Model file for the job. Use its own axes, mm. Face numbers are marked on the shaded views. A direction names the side the tool comes from. Coordinates: 2 decimals unless noted, no trailing zeros. Loops run counter-clockwise (first coordinate to the right, second up) from the corner with the lowest first, then second, coordinate; pieces in that order, holes last. Notation, with made-up numbers: (72, -24) -> (91, -24) arc R22 ccw to (91, -2) -> close; hole circle Ø8 at (88, 46). An arc over 180 degrees is marked (long way). Use one line per item in the form item = value.
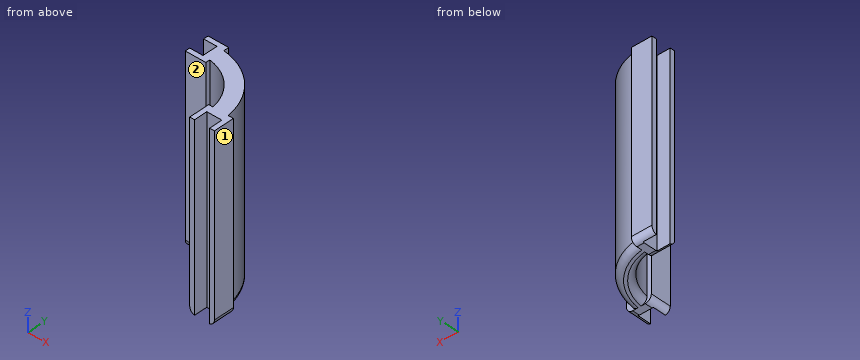
```python
from build123d import *

# Parameters (mm, degrees)
EXTRUDE_1_DEPTH = 150
EXTRUDE_2_DEPTH = 150
FILLET_1_R      = 5
FILLET_2_R      = 5
FILLET_3_R      = 5
FILLET_4_R      = 5
FILLET_5_R      = 5


with BuildPart() as part:
    # 草图1 → 凸台-拉伸1 (new body)
    with BuildSketch(Plane.XY):
        with BuildLine():
            Line((0, 40), (0, 52.5))
            ThreePointArc((0, 52.5), (37.123106012, 37.123106012), (52.5, 0))
            Line((52.5, 0), (40, 0))
            ThreePointArc((40, 0), (28.284271247, 28.284271247), (0, 40))
        make_face()
    extrude(amount=EXTRUDE_1_DEPTH)

    # 草图2 → 凸台-拉伸2 (add)
    with BuildSketch(Plane(origin=(0, 0, 0), x_dir=(-1, 0, 0), z_dir=(0, 0, -1))):
        Polygon((11, 52.5), (11, 56.5), (-6.040960951, 56.5), (-6.040960951, 36), (11, 36), (11, 40), (0, 40), (0, 52.5), align=None)
        Polygon((-52.5, -11), (-52.5, 0), (-40, 0), (-40, -11), (-36, -11), (-36, 6.040960951), (-56.5, 6.040960951), (-56.5, -11), align=None)
    extrude(amount=-EXTRUDE_2_DEPTH)

    # 圆角1
    fillet_1_edges = [part.edges().sort_by_distance(p)[0] for p in [
        (37.123106012, 37.123106012, 0),
    ]]
    fillet(fillet_1_edges, radius=FILLET_1_R)

    # 圆角2
    # the kernel refuses this fillet: 5 mm, written as the material it takes off along each edge
    with BuildSketch(Plane(origin=(0, 0, 0), x_dir=(0.9870710552033948, -0.1602832866510314, 0), z_dir=(-0.1602832866510314, -0.9870710552033948, 0))) as fillet_2_piece_1_section:
        with BuildLine():
            CenterArc((40 + FILLET_2_R, FILLET_2_R), FILLET_2_R, 180, 90)
            Line((40, FILLET_2_R), (40, 0))
            Line((40, 0), (40 + FILLET_2_R, 0))
        make_face()
    fillet_2_piece_1 = revolve(axis=Axis((0, 0, 0), (0, 0, 1)), revolution_arc=108.446679136, mode=Mode.PRIVATE)
    fillet_2_piece_1 = split(fillet_2_piece_1, bisect_by=Plane(origin=(6.040960951, 29.285093623, 1.415376577), z_dir=(1, 0, 0)), keep=Keep.TOP, mode=Mode.PRIVATE)
    fillet_2_piece_1 = split(fillet_2_piece_1, bisect_by=Plane(origin=(29.285093623, 6.040960951, 1.415376577), z_dir=(0, 1, 0)), keep=Keep.TOP, mode=Mode.PRIVATE)
    add(fillet_2_piece_1, mode=Mode.SUBTRACT)

    # 圆角3
    fillet_3_edges = [part.edges().sort_by_distance(p)[0] for p in [
        (-2.479519525, 56.5, 0),
    ]]
    fillet(fillet_3_edges, radius=FILLET_3_R)

    # 圆角4
    fillet_4_edges = [part.edges().sort_by_distance(p)[0] for p in [
        (56.5, -2.479519525, 0),
        (-2.479519525, 36, 0),
    ]]
    fillet(fillet_4_edges, radius=FILLET_4_R)

    # 圆角5
    fillet_5_edges = [part.edges().sort_by_distance(p)[0] for p in [
        (36, -2.479519525, 0),
    ]]
    fillet(fillet_5_edges, radius=FILLET_5_R)


solid = part.part
```
Q1. Band-saw the part on A-A, the plane x = -4.5. Write the cut outline in (y, z), and give its area (3 significant figures).
Result:
outline = (36, 5) arc R5 ccw to (40, 0.1) -> (40, 150) -> (36, 150) -> close; (52.5, 0.1) arc R5 ccw to (56.5, 5) -> (56.5, 150) -> (52.5, 150) -> close
area = 1,190 mm2
Q2. Which spindle directions (+Z, -Z, +X, -X, +Y, -Y) get a long thin tool onto all of the face, cutting with end or side? Do the marked faces 1 and 2. Say none if no direction does.
Result:
face_1 = +Z, -Z, +X, +Y, -Y
face_2 = +Z, -Z, -X, -Y
Q3. Band-saw the part on B-B, the plane z = 103.5. Write the cut outline in (x, y), and give its area (3 significant figures).
Result:
outline = (-11, 36) -> (6.04, 36) -> (6.04, 39.54) arc R40 cw to (39.54, 6.04) -> (36, 6.04) -> (36, -11) -> (40, -11) -> (40, 0) -> (52.5, 0) -> (52.5, -11) -> (56.5, -11) -> (56.5, 6.04) -> (52.15, 6.04) arc R52.5 ccw to (6.04, 52.15) -> (6.04, 56.5) -> (-11, 56.5) -> (-11, 52.5) -> (0, 52.5) -> (0, 40) -> (-11, 40) -> close
area = 1,180 mm2
Q4. Wall check: line 1 along Y through (x, z) = (-7, 38.5); line 2 along X through (y, z) = (2, 66). Give the ranges that are in metal, low to high.
Result:
line_1 = 36 to 40, 52.5 to 56.5
line_2 = 36 to 56.5
Q5. Pin check, flat tips, straight feed: pin 1 Ø8.5 at (x, z) = (1, 43.5) entering from -Y; pin 2 Ø5.5 at (y, z) = (-3, 63) entering from -X; pin 3 Ø5 at (y, z) = (27, 30.5) entering from -X. Stop position of each tip, or through.
Result:
pin_1 = 36
pin_2 = 36
pin_3 = 27.01
